```python
from build123d import *

# Parameters (mm, degrees)
ESBO_O1_R                = 1.6
ESBO_O1_R_2              = 2
ESBO_O1_W                = 31
ESBO_O1_H                = 9
RESSALTO_EXTRUS_O1_DEPTH = 3


with BuildPart() as part:
    # Esboço1 → Ressalto-extrusão1 (new body)
    with BuildSketch(Plane.XY):
        Polygon((-94, -9.5), (-94, -15), (94, -15), (94, -9.5), (100, -9.5), (100, 0), (94, 0), (94, 15), (-94, 15), (-94, 0), (-100, 0), (-100, -9.5), align=None)
        with Locations((-97, -4.75)):
            Circle(ESBO_O1_R, mode=Mode.SUBTRACT)
        with Locations((97, -4.75)):
            Circle(ESBO_O1_R, mode=Mode.SUBTRACT)
        with Locations((-74, 0)):
            Circle(ESBO_O1_R_2, mode=Mode.SUBTRACT)
        with Locations((-37.4, 0)):
            Circle(ESBO_O1_R_2, mode=Mode.SUBTRACT)
        with Locations((37.4, 0)):
            Circle(ESBO_O1_R_2, mode=Mode.SUBTRACT)
        with Locations((74, 0)):
            Circle(ESBO_O1_R_2, mode=Mode.SUBTRACT)
        with Locations((-55.7, 0)):
            Rectangle(ESBO_O1_W, ESBO_O1_H, mode=Mode.SUBTRACT)
        with Locations((55.7, 0)):
            Rectangle(ESBO_O1_W, ESBO_O1_H, mode=Mode.SUBTRACT)
    extrude(amount=RESSALTO_EXTRUS_O1_DEPTH)


solid = part.part
```
Part model, mm, in its own coordinate system. Round coordinates to 2 decimals unless told otherwise and drop trailing zeros. Order: outer loops, then holes, each group sorted by start corner. A loop starts at its lowest first (then second) coordinate and runs counter-clockwise, first axis right, second up. Notation, with made-up numbers: M -33.5,-6.5 L -14.5,-6.5 A22 cw -14.5,27.5 Z; hole C 55.5,16.5 d11. An arc over 180 degrees is marked long. Put each result on its own line as item: value. Start each with the question number.
1. Drill centre lines: probe 1 along Y at (x, z) = (-37.4, 2.2); probe 2 along Y at (x, z) = (-45, 2.6); probe 3 along X at (y, z) = (9, 0.7). Where is each one in solid material? Low to high. Write a range as [from, to].
2. Drop flat-ended pins along their axis: pin 1 (5 mm diameter, centred on x = -25.5, y = -10.5, fed in from -Z); pin 2 (0.9 mm diameter, centred on y = 2, z = 1, fed in from -X). Give the stop position or say it passes through.
3. Slice it at A-A on x = -74. List the corners of the cut face in (y, z), then the cut area to 3 significant figures.
4. Slice it at D-D on y = -12.25. List the corners of the cut face in (x, z).
5. Two-plate mould, pull along X, no slides. Class faces 1 (the face through (-1, 0, 0)), 2 (the face through (35.402, 0.088, 1.479)): +X half, -X half, draft (parallel to the pull), parting line (faces both ways), or undercut.
6. Slice it at B-B on z = 0.5. State how many separate pieces and enclosed holes the cut face has, then the cut area to 3 significant figures.
7. Slice it at C-C on x = 66.5. List the corners of the cut face in (y, z).
Findings:
1. probe 1: [-15, -2], [2, 15]
1. probe 2: [-15, -4.5], [4.5, 15]
1. probe 3: [-94, 94]
2. pin 1: z = 0
2. pin 2: x = -94
3. outline: M -15,0 L -2,0 L -2,3 L -15,3 Z; M 2,0 L 15,0 L 15,3 L 2,3 Z
3. area: 78.0 mm2
4. outline: M -94,0 L 94,0 L 94,3 L -94,3 Z
5. face 1: draft
5. face 2: undercut
6. separate pieces: 1
6. enclosed holes: 8
6. area: 5,130 mm2
7. outline: M -15,0 L -4.5,0 L -4.5,3 L -15,3 Z; M 4.5,0 L 15,0 L 15,3 L 4.5,3 Z
